Check sheet for the modelled part. Datum: model origin and axes. Units: mm. Face numbers are marked on the shaded views. Give positions to 0.01 mm unless a question says otherwise; leave off trailing zeros. Loops run counter-clockwise (first coordinate to the right, second up) from the corner with the lowest first, then second, coordinate; pieces in that order, holes last. Notation, with made-up numbers: M 43.25,83 L 73.25,83 A12 ccw 73.25,87 Z; hole C 31.5,-34.5 d9. An arc over 180 degrees is marked long. Use one line per item in the form item = value.
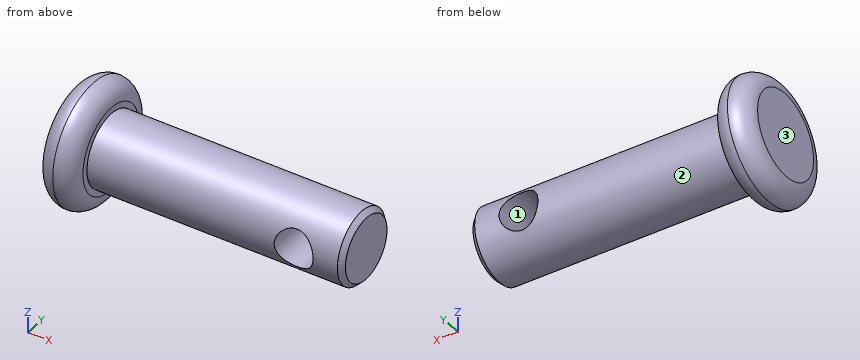
from build123d import *

# Parameters (mm, degrees)
SKETCH_2_R          = 0.8
CUT_EXTRUDE_1_DEPTH = 10
CHAMFER_1_SIZE      = 0.2
FILLET_1_R          = 0.75


with BuildPart() as part:
    # 草图1 → 旋转1 (revolve)
    with BuildSketch(Plane.XY):
        Polygon((0, 0), (0, 2.5), (1.5, 2.5), (1.5, 1.5), (12, 1.5), (12, 0), align=None)
    revolve(axis=Axis((12, 0, 0), (-1, 0, 0)))

    # 草图2 → 切除-拉伸1 (cut, symmetric)
    with BuildSketch(Plane(origin=(0, 0, 0), x_dir=(1, 0, 0), z_dir=(0, 1, 0))):
        with Locations(Location((10, 0, 0), (0, 0, 270))):
            Circle(SKETCH_2_R)
    extrude(amount=CUT_EXTRUDE_1_DEPTH, both=True, mode=Mode.SUBTRACT)

    # 倒角1
    chamfer_1_edges = [part.edges().sort_by_distance(p)[0] for p in [
        (12, -1.5, 0),
    ]]
    chamfer(chamfer_1_edges, length=CHAMFER_1_SIZE)

    # 圆角1
    fillet_1_edges = [part.edges().sort_by_distance(p)[0] for p in [
        (1.5, -2.5, 0),
        (0, -2.5, 0),
    ]]
    fillet(fillet_1_edges, radius=FILLET_1_R - 0.0001)  # a hair under: the kernel refuses the full size


solid = part.part
1) Release check for a two-part mould opening along Z. For the marked faces 1, 2 and 3 record: pulls with the +Z half, pulls with the -Z half, needs draft (parallel to the pull), parting line crosses it, or undercut.
Evaluation:
face_1 = undercut
face_2 = parting line crosses it
face_3 = needs draft
2) Depth check by flat-ended pin: pin 1 Ø3 at (x, z) = (2.5, 0) entering from +Y; pin 2 Ø1.8 at (x, z) = (10, 0) entering from +Y; pin 3 Ø3 at (x, z) = (3, 2) entering from -Y. Enter the tip coordinate at first touch or a pass-through.
Evaluation:
pin_1 = 2.46
pin_2 = 1.5
pin_3 = -1.41
3) Scan lines: line 1 (X direction, y = -0.1, z = 0); line 2 (X direction, y = 0.45, z = 0.3); line 3 (Z direction, x = 10.5, y = -1.25). Record each from-to range of solid material in increasing order.
Evaluation:
line_1 = 0 to 9.2, 10.8 to 12
line_2 = 0 to 9.26, 10.74 to 12
line_3 = -0.83 to -0.62, 0.62 to 0.83
4) Section check C-C (x = 10). Record the cut outline in (y, z), then the cut area to 3 significant figures.
Evaluation:
outline = M -1.27,-0.8 A1.5 ccw 1.27,-0.8 Z; M -1.27,0.8 L 1.27,0.8 A1.5 ccw Z
area = 2.51 mm^2
5) Section check B-B (x = 8.75). Record the cut outline in (y, z), then the cut area to 3 significant figures.
Evaluation:
outline = C 0,0 d3
area = 7.07 mm^2
